from build123d import *

# Parameters (mm, degrees)
SKETCH1_R               = 2.5
BOSS_EXTRUDE1_DEPTH     = 3
BOSS_EXTRUDE2_DEPTH     = 23
FILLET1_R               = 13
FILLET2_R               = 8
SKETCH2_R               = 4
CUT_EXTRUDE1_DEPTH      = 39.499999627
CUT_EXTRUDE1_DEPTH_BACK = 92.500000373
SKETCH3_R               = 2.25
CUT_EXTRUDE2_DEPTH      = 34.083768895
CUT_EXTRUDE2_DEPTH_BACK = 62.916231105


with BuildPart() as part:
    # Sketch1 → Boss-Extrude1 (new body)
    with BuildSketch(Plane(origin=(0, 0, 0), x_dir=(0, 0, -1), z_dir=(1, 0, 0))):
        with BuildLine():
            ThreePointArc((47.5, 54.5), (44.424621202, 61.924621202), (37, 65))
            Line((37, 65), (-37, 65))
            ThreePointArc((-37, 65), (-44.424621202, 61.924621202), (-47.5, 54.5))
            Line((-47.5, 54.5), (-47.5, 20.500000268))
            ThreePointArc((-47.5, 20.500000268), (-44.424621202, 13.075379066), (-37, 10.000000268))
            Line((-37, 10.000000268), (-11.583769402, 10.000000268))
            Line((-11.583769402, 10.000000268), (-11.583769402, -8.500000373))
            Line((-11.583769402, -8.500000373), (-37, -8.500000373))
            ThreePointArc((-37, -8.500000373), (-44.424621202, -11.57537917), (-47.5, -19.000000373))
            Line((-47.5, -19.000000373), (-47.5, -54.5))
            ThreePointArc((-47.5, -54.5), (-44.424621202, -61.924621202), (-37, -65))
            Line((-37, -65), (37, -65))
            ThreePointArc((37, -65), (44.424621202, -61.924621202), (47.5, -54.5))
            Line((47.5, -54.5), (47.5, -19.000000373))
            ThreePointArc((47.5, -19.000000373), (44.424621202, -11.57537917), (37, -8.500000373))
            Line((37, -8.500000373), (11.416231668, -8.500000373))
            Line((11.416231668, -8.500000373), (11.416231668, 10.000000268))
            Line((11.416231668, 10.000000268), (37, 10.000000268))
            ThreePointArc((37, 10.000000268), (44.424621202, 13.075379066), (47.5, 20.500000268))
            Line((47.5, 20.500000268), (47.5, 54.5))
        make_face()
        with Locations((-35, -34.75)):
            Circle(SKETCH1_R, mode=Mode.SUBTRACT)
        with Locations((35, -34.75)):
            Circle(SKETCH1_R, mode=Mode.SUBTRACT)
        with Locations((-35, 34.75)):
            Circle(SKETCH1_R, mode=Mode.SUBTRACT)
        with Locations((35, 34.75)):
            Circle(SKETCH1_R, mode=Mode.SUBTRACT)
    extrude(amount=BOSS_EXTRUDE1_DEPTH)

    # Sketch1_3 → Boss-Extrude2 (add)
    with BuildSketch(Plane(origin=(0, 0, 0), x_dir=(0, 0, -1), z_dir=(1, 0, 0))):
        Polygon((-36.583768839, 10.000000268), (-36.583768839, 28.000000268), (-14.583768839, 28.000000268), (-14.583768839, 41.000000268), (-10.33376912, 41.000000268), (-10.33376912, -39.500000373), (-14.583768839, -39.500000373), (-14.583768839, -26.500000373), (-36.583768839, -26.500000373), (-36.583768839, -8.500000373), (-23.615095491, -8.500000373), (-11.583769402, -8.500000373), (-11.583769402, 10.000000268), (-23.615095491, 10.000000268), align=None)
        Polygon((11.416231668, -8.500000373), (11.416231668, 10.000000268), (23.447557757, 10.000000268), (36.416231105, 10.000000268), (36.416231105, 28.000000268), (14.416231105, 28.000000268), (14.416231105, 41.000000268), (10.166231386, 41.000000268), (10.166231386, -39.500000373), (14.416231105, -39.500000373), (14.416231105, -26.500000373), (36.416231105, -26.500000373), (36.416231105, -8.500000373), (23.447557757, -8.500000373), align=None)
    extrude(amount=BOSS_EXTRUDE2_DEPTH)

    # Fillet1
    fillet1_edges = [part.edges().sort_by_distance(p)[0] for p in [
        (23, 19.000000268, -36.416231105),
        (23, -17.500000373, -36.416231105),
        (23, 19.000000268, 36.583768839),
        (23, -17.500000373, 36.583768839),
    ]]
    fillet(fillet1_edges, radius=FILLET1_R)

    # Fillet2
    fillet2_edges = [part.edges().sort_by_distance(p)[0] for p in [
        (23, 41.000000268, -12.291231246),
        (23, -39.500000373, -12.291231246),
        (23, -39.500000373, 12.45876898),
        (23, 41.000000268, 12.45876898),
    ]]
    fillet(fillet2_edges, radius=FILLET2_R)

    # Sketch2 → Cut-Extrude1 (cut, two sides)
    with BuildSketch(Plane.XZ.offset(26.500000373)) as cut_extrude1_sk:
        with Locations((9.5, 28.083768839)):
            Circle(SKETCH2_R)
        with Locations((9.5, -28.083768839)):
            Circle(SKETCH2_R)
    extrude(amount=CUT_EXTRUDE1_DEPTH, mode=Mode.SUBTRACT)
    extrude(cut_extrude1_sk.sketch, amount=-CUT_EXTRUDE1_DEPTH_BACK, mode=Mode.SUBTRACT)

    # Sketch3 → Cut-Extrude2 (cut, two sides)
    with BuildSketch(Plane(origin=(0, 0, -14.416231105), x_dir=(-1, 0, 0), z_dir=(0, 0, -1))) as cut_extrude2_sk:
        with Locations((-13, -33.000000373)):
            Circle(SKETCH3_R)
        with Locations((-13, 33.000000373)):
            Circle(SKETCH3_R)
    extrude(amount=CUT_EXTRUDE2_DEPTH, mode=Mode.SUBTRACT)
    extrude(cut_extrude2_sk.sketch, amount=-CUT_EXTRUDE2_DEPTH_BACK, mode=Mode.SUBTRACT)


solid = part.part
Could you check a few things on this model? Use its own coordinates, in mm. A direction names the side the tool comes from. Round coordinates to 2 decimals unless told otherwise and drop trailing zeros. Order: outer loops, then holes, each group sorted by start corner. A loop starts at its lowest first (then second) coordinate and runs counter-clockwise, first axis right, second up. Notation, with made-up numbers: M -11,62.25 L 13,62.25 A21 cw 13,99.25 Z; hole C 82.5,74 d6. An arc over 180 degrees is marked long. One line per item, written item: value.
(1) Imagine slicing it at B-B (x = 19). Write out the boundary of the cut face in (y, z), and give its area (3 significant figures).
Ans:
outline: M -38.43,-14.42 L -26.5,-14.42 L -26.5,-32.8 L -8.5,-32.8 L -8.5,-11.42 L 10,-11.42 L 10,-32.8 L 28,-32.8 L 28,-14.42 L 39.93,-14.42 L 39.93,-10.17 L -38.43,-10.17 Z; M -38.43,10.33 L 39.93,10.33 L 39.93,14.58 L 28,14.58 L 28,32.96 L 10,32.96 L 10,11.58 L -8.5,11.58 L -8.5,32.96 L -26.5,32.96 L -26.5,14.58 L -38.43,14.58 Z
area: 1,880 mm^2
(2) I need wall thicknesses on line 1 along Y through (x, z) = (1.8, 35); line 2 along Z through (x, y) = (9.5, 19.25); line 3 along Y through (x, z) = (13.5, 19). Which ranges of each line are inside material? Lowest first, please. Write a range as from..to.
Ans:
line 1: y = -65..-37.25, -32.25..-8.5, 10..32.25, 37.25..65
line 2: z = -36.42..-32.08, -24.08..-10.17, 10.33..24.08, 32.08..36.58
line 3: y = -26.5..-8.5, 10..28
(3) If we mould it in two halves opening along Z, with no side actions, what happens to faces 1 (the flat face through (13, 1, -10.166)), 2 (the flat face through (11, 10, 24)), 3 (the cylindrical face through (5.504, 18.874, 28.26)), 4 (the flat face through (13, 36, 14.584))? For each: released by +Z, released by -Z, zero draft, split by the parting line, or undercut.
Ans:
face 1: undercut
face 2: zero draft
face 3: undercut
face 4: released by +Z
(4) I'm going to push flat-ended pins straight in: P1, Ø4.5, axis at x = 9.5, z = 13, coming from the +Y side; P2, Ø3, axis at y = 13.5, z = 26, coming from the +X side; P3, Ø1.5, axis at y = 33.5, z = -24.5, coming from the +X side; P4, Ø5, axis at x = 9.5, z = -28.08, coming from the +Y side. Where does each tip first touch, or does it pass through?
Ans:
P1: stops at y = 41
P2: stops at x = 22.97
P3: stops at x = 3
P4: passes through
(5) Imagine slicing it at C-C (z = 35). Write out the boundary of the cut face in (x, y), and give its area (3 significant figures).
Ans:
outline: M 0,-65 L 3,-65 L 3,-37.25 L 0,-37.25 Z; M 0,-32.25 L 3,-32.25 L 3,-26.5 L 16.22,-26.5 L 16.22,-8.5 L 0,-8.5 Z; M 0,10 L 16.22,10 L 16.22,28 L 3,28 L 3,32.25 L 0,32.25 Z; M 0,37.25 L 3,37.25 L 3,65 L 0,65 Z
area: 780 mm^2
(6) Imagine slicing it at D-D (y = 11.5). Write out the boundary of the cut face in (x, z), and give its area (3 significant figures).
Ans:
outline: M 0,-42.41 L 3,-42.41 L 3,-36.42 L 10,-36.42 A13 ccw 23,-23.42 L 23,-10.17 L 3,-10.17 L 3,10.33 L 23,10.33 L 23,23.58 A13 ccw 10,36.58 L 3,36.58 L 3,42.41 L 0,42.41 Z; hole C 9.5,-28.08 d8; hole C 9.5,28.08 d8
area: 1,130 mm^2
(7) Imagine slicing it at A-A (z = -18). Write out the boundary of the cut face in (x, y).
Ans:
outline: M 0,-65 L 3,-65 L 3,-26.5 L 23,-26.5 L 23,-8.5 L 0,-8.5 Z; M 0,10 L 23,10 L 23,28 L 3,28 L 3,65 L 0,65 Z
(8) Which directions (+Z, -Z, +X, -X, +Y, -Y) give clear straight access to the entire face, cutting with the end or side of a thin tool? Please do faces 5 (the flat face through (11, -8.5, 24)), 6 (the flat face through (11, 10, -24)), 7 (the flat face through (9, -39.5, -12)), 8 (the flat face through (13, -26.5, 25)).
Ans:
face 5: +Z, +X, -X
face 6: -Z, +X, -X
face 7: +Z, -Z, +X, -Y
face 8: +Z, +X, -Y
